from build123d import *

# Parameters (mm, degrees)
ESQUISSE1_W                                        = 53.8
ESQUISSE1_H                                        = 51.7
ESQUISSE1_R                                        = 1.1
BOSS_EXTRU_1_DEPTH                                 = 3
CHAMBRAGE_POUR_VIS_SIX_PANS_CREUX_M1_6_D           = 2.2
CHAMBRAGE_POUR_VIS_SIX_PANS_CREUX_M1_6_CBORE_D     = 3.8
CHAMBRAGE_POUR_VIS_SIX_PANS_CREUX_M1_6_CBORE_DEPTH = 1.2
BOSS_EXTRU_2_START                                 = 16
ESQUISSE4_W                                        = 7.51
ESQUISSE4_H                                        = 51.7
BOSS_EXTRU_2_DEPTH                                 = 19
ESQUISSE6_R                                        = 1.6
ENL_V_MAT_EXTRU_2_DEPTH                            = 62.22146764
CHAMBRAGE_POUR_VIS_SIX_PANS_CREUX_M31_D            = 3.2
CHAMBRAGE_POUR_VIS_SIX_PANS_CREUX_M31_CBORE_D      = 6.5
CHAMBRAGE_POUR_VIS_SIX_PANS_CREUX_M31_CBORE_DEPTH  = 7
ENL_V_MAT_EXTRU_3_DEPTH                            = 77.075175977
ENL_V_MAT_EXTRU_3_DEPTH_BACK                       = 77.075175977
BOSS_EXTRU_3_DEPTH                                 = 2
CHANFREIN1_SIZE                                    = 2


with BuildPart() as part:
    # Esquisse1 → Boss.-Extru.1 (new body)
    with BuildSketch(Plane(origin=(0, 0, 0), x_dir=(1, 0, 0), z_dir=(0, 1, 0))):
        with Locations((16.5, -2.35)):
            Rectangle(ESQUISSE1_W, ESQUISSE1_H)
        with Locations(Location((12.3, -25.2, 0), (0, 0, 270))):
            Circle(ESQUISSE1_R, mode=Mode.SUBTRACT)
        with BuildLine():
            ThreePointArc((13.170256267, -22.2), (-7.69, -14.95), (13.170256267, -7.7))
            Line((13.170256267, -7.7), (38.4, -7.7))
            Line((38.4, -7.7), (38.4, -22.2))
            Line((38.4, -22.2), (13.170256267, -22.2))
        make_face(mode=Mode.SUBTRACT)
        with Locations(Location((12.3, -4.7, 0), (0, 0, 270))):
            Circle(ESQUISSE1_R, mode=Mode.SUBTRACT)
        with Locations(Location((33, -25.2, 0), (0, 0, 270))):
            Circle(ESQUISSE1_R, mode=Mode.SUBTRACT)
        with Locations(Location((33, -4.7, 0), (0, 0, 270))):
            Circle(ESQUISSE1_R, mode=Mode.SUBTRACT)
        with Locations(Location((0, 0, 0), (0, 0, 270))):
            Circle(ESQUISSE1_R, mode=Mode.SUBTRACT)
        with Locations(Location((0, 20.5, 0), (0, 0, 270))):
            Circle(ESQUISSE1_R, mode=Mode.SUBTRACT)
        with Locations(Location((20.7, 0, 0), (0, 0, 270))):
            Circle(ESQUISSE1_R, mode=Mode.SUBTRACT)
        with BuildLine():
            Line((-5.4, 3), (-5.4, 17.5))
            Line((-5.4, 17.5), (19.829743733, 17.5))
            ThreePointArc((19.829743733, 17.5), (32.837694897, 21.29211021), (40.69, 10.25))
            ThreePointArc((40.69, 10.25), (32.837694897, -0.79211021), (19.829743733, 3))
            Line((19.829743733, 3), (-5.4, 3))
        make_face(mode=Mode.SUBTRACT)
        with Locations(Location((20.7, 20.5, 0), (0, 0, 270))):
            Circle(ESQUISSE1_R, mode=Mode.SUBTRACT)
    extrude(amount=BOSS_EXTRU_1_DEPTH)

    # Chambrage pour vis à six pans creux M1.61 (through all)
    with Locations(Plane(origin=(0, 3, 0), x_dir=(1, 0, 0), z_dir=(0, 1, 0))):
        with Locations((0, 20.5), (20.7, 20.5), (20.7, 0), (12.3, -4.7), (0, 0), (33, -4.7), (12.3, -25.2), (33, -25.2)):
            CounterBoreHole(CHAMBRAGE_POUR_VIS_SIX_PANS_CREUX_M1_6_D / 2, CHAMBRAGE_POUR_VIS_SIX_PANS_CREUX_M1_6_CBORE_D / 2, CHAMBRAGE_POUR_VIS_SIX_PANS_CREUX_M1_6_CBORE_DEPTH)

    # Esquisse4 → Boss.-Extru.2 (add)
    with BuildSketch(Plane.XZ.offset(BOSS_EXTRU_2_START)):
        with BuildLine():
            Line((-6.31, 28.2), (-10.4, 28.2))
            Line((-10.4, 28.2), (-10.4, -23.5))
            Line((-10.4, -23.5), (-6.31, -23.5))
            Line((-6.31, -23.5), (-6.31, 9.440009074))
            ThreePointArc((-6.31, 9.440009074), (-7.69, 14.95), (-6.31, 20.459990926))
            Line((-6.31, 20.459990926), (-6.31, 28.2))
        make_face()
        with Locations((-14.155, 2.35)):
            Rectangle(ESQUISSE4_W, ESQUISSE4_H)
        with BuildLine():
            Line((39.31, 28.2), (50.91, 28.2))
            Line((50.91, 28.2), (50.91, -23.5))
            Line((50.91, -23.5), (39.31, -23.5))
            Line((39.31, -23.5), (39.31, -15.759990926))
            ThreePointArc((39.31, -15.759990926), (40.69, -10.25), (39.31, -4.740009074))
            Line((39.31, -4.740009074), (39.31, 28.2))
        make_face()
    extrude(amount=-BOSS_EXTRU_2_DEPTH)

    # Esquisse6 → Enlèv. mat.-Extru.2 (cut, through all)
    with BuildSketch(Plane(origin=(0, 3, 0), x_dir=(1, 0, 0), z_dir=(0, 1, 0))):
        with Locations(Location((-12.11, 15.5, 0), (0, 0, 270))):
            Circle(ESQUISSE6_R)
        with Locations(Location((-12.11, -20.2, 0), (0, 0, 90))):
            Circle(ESQUISSE6_R)
        with Locations(Location((45.11, -20.2, 0), (0, 0, 270))):
            Circle(ESQUISSE6_R)
        with Locations(Location((45.11, 15.5, 0), (0, 0, 90))):
            Circle(ESQUISSE6_R)
    extrude(amount=-ENL_V_MAT_EXTRU_2_DEPTH, mode=Mode.SUBTRACT)

    # Chambrage pour vis à six pans creux M31 (through all)
    with Locations(Plane(origin=(0, 3, 0), x_dir=(1, 0, 0), z_dir=(0, 1, 0))):
        with Locations((-12.11, 15.5), (-12.11, -20.2), (45.11, 15.5), (45.11, -20.2)):
            CounterBoreHole(CHAMBRAGE_POUR_VIS_SIX_PANS_CREUX_M31_D / 2, CHAMBRAGE_POUR_VIS_SIX_PANS_CREUX_M31_CBORE_D / 2, CHAMBRAGE_POUR_VIS_SIX_PANS_CREUX_M31_CBORE_DEPTH)

    # Esquisse9 → Enlèv. mat.-Extru.3 (cut, two sides: drawn at the far end of the back side and taken through both)
    with BuildSketch(Plane.ZY.offset(17.91).offset(-ENL_V_MAT_EXTRU_3_DEPTH_BACK)):
        Polygon((-23.5, -8.5), (-8.5, -8.5), (-2.65, -3), (7.35, -3), (13.2, -8.5), (28.2, -8.5), (28.2, -16), (-23.5, -16), align=None)
    extrude(amount=ENL_V_MAT_EXTRU_3_DEPTH + ENL_V_MAT_EXTRU_3_DEPTH_BACK, mode=Mode.SUBTRACT)

    # Esquisse10 → Boss.-Extru.3 (add)
    with BuildSketch(Plane.XY.offset(28.2)):
        Polygon((-6.31, -8.5), (-1.905, -4.25), (34.905, -4.25), (39.31, -8.5), (50.91, -8.5), (50.91, 3), (-17.91, 3), (-17.91, -8.5), align=None)
    boss_extru_3 = extrude(amount=BOSS_EXTRU_3_DEPTH)

    # Symétrie1: Boss.-Extru.3 across plane
    add(boss_extru_3.mirror(Plane.XY.offset(2.35)))

    # Chanfrein1
    chanfrein1_edges = [part.edges().sort_by_distance(p)[0] for p in [
        (-17.91, 3, 2.35),
        (50.91, 3, 2.35),
        (50.91, -2.75, 30.2),
        (16.5, 3, 30.2),
        (-17.91, -2.75, 30.2),
        (-17.91, -2.75, -25.5),
        (16.5, 3, -25.5),
        (50.91, -2.75, -25.5),
    ]]
    chamfer(chanfrein1_edges, length=CHANFREIN1_SIZE)


solid = part.part
Verification items for the finished model (mm, model axes). A direction names the side the tool comes from. Coordinates: 2 decimals unless noted, no trailing zeros. Order: outer loops, then holes, each group sorted by start corner. A loop starts at its lowest first (then second) coordinate and runs counter-clockwise, first axis right, second up. Notation, with made-up numbers: M 53,67.25 L 82,67.25 A9 ccw 82,80.25 Z; hole C 49.5,62 d10. An arc over 180 degrees is marked long. One line per item, written item: value. Start each with the question number.
Item 1: Sectioned sample at C-C (x = 16.5). Enter the section's corners in (y, z), then the cut area to 3 significant figures.
Item 2: Sectioned sample at A-A (y = -5.75). Count the separate pieces of the cut face and the enclosed holes in it, then the cut area to 3 significant figures.
Item 3: Scan lines: probe 1 along Z at (x, y) = (45, -1.5); probe 2 along Z at (x, y) = (-3, -3.75); probe 3 along Z at (x, y) = (15, 0.75). Record each from-to range of solid material in increasing order.
Item 4: Sectioned sample at B-B (z = -10.25). Enter the section's corners in (x, y), then the cut area to 3 significant figures.
Item 5: Access from +Z, -Z, +X, -X, +Y, -Y to the whole of each face (thin tool, end or side, straight path). Record for faces 1 (the flat face through (26, 1, 7.7)), 2 (the flat face through (16, -4.25, -24)), 3 (the flat face through (45, -3, 2)), 4 (the cylindrical face through (-9.01, -0.45, 19.22)), 5 (the flat face through (-13, -8.5, 22)).
Item 6: Sectioned sample at D-D (y = -1.5). Enter the section's corners in (x, z), then the cut area to 3 significant figures.
Item 7: Gauge pin test, flat ends, axial feed: pin 1 (1 mm diameter, centred on y = -5, z = -1.5, fed in from +X); pin 2 (1.1 mm diameter, centred on x = 33, z = 4, fed in from +Y); pin 3 (12 mm diameter, centred on x = 14.5, z = -16.5, fed in from -Y). Record the tip position at first contact, or that the pin passes through.
Item 8: Mould release check, pull along X, two halves, no side actions. Record for faces 6 (the flat face through (49.542, 1.604, 28.964)), 7 (the flat face through (-4.138, -6.405, 29.186)), 8 (the flat face through (17, 3, 3)): released by +X, released by -X, zero draft, split by the parting line, or undercut.
Conclusion:
1. outline: M -4.25,-25.5 L 1,-25.5 L 3,-23.5 L 3,-17.5 L 0,-17.5 L 0,-23.5 L -4.25,-23.5 Z; M -4.25,28.2 L 0,28.2 L 0,22.2 L 3,22.2 L 3,28.2 L 1,30.2 L -4.25,30.2 Z; M 0,-3 L 3,-3 L 3,7.7 L 0,7.7 Z
1. area: 93.1 mm^2
2. separate pieces: 4
2. enclosed holes: 4
2. area: 887 mm^2
3. probe 1: z = -25.5 to -18.75, -12.25 to 16.95, 23.45 to 30.2
3. probe 2: z = -25.5 to -23.5, 28.2 to 30.2
3. probe 3: z = -25.5 to -17.5, -3 to 7.7, 22.2 to 30.2
4. outline: M -17.91,-8.5 L -6.31,-8.5 L -6.31,0 L -5.4,0 L -5.4,3 L -15.91,3 L -17.91,1 Z; M 40.69,-8.5 L 50.91,-8.5 L 50.91,1 L 48.91,3 L 40.69,3 Z
4. area: 250 mm^2
5. face 1: +Y, -Y
5. face 2: +Z, -Z, -Y
5. face 3: +X, -X, -Y
5. face 4: +Y
5. face 5: +Z, -Z, +X, -X, -Y
6. outline: M -17.91,-23.5 L -15.91,-25.5 L 48.91,-25.5 L 50.91,-23.5 L 50.91,28.2 L 48.91,30.2 L -15.91,30.2 L -17.91,28.2 Z; hole C -12.11,-15.5 d6.5; hole C -12.11,20.2 d6.5; hole M -6.31,-23.5 L 39.31,-23.5 L 39.31,-15.76 A11.69 ccw 39.31,-4.74 L 39.31,28.2 L -6.31,28.2 L -6.31,20.46 A11.69 ccw -6.31,9.44 Z; hole C 45.11,-15.5 d6.5; hole C 45.11,20.2 d6.5
6. area: 1,310 mm^2
7. pin 1: passes through
7. pin 2: stops at y = 1.8
7. pin 3: stops at y = 0
8. face 6: released by +X
8. face 7: undercut
8. face 8: zero draft
